Can you work these out from the model? Positions are in its coordinate system, mm. A direction names the side the tool comes from. Give positions to 0.01 mm unless a question says otherwise; leave off trailing zeros. Loops run counter-clockwise (first coordinate to the right, second up) from the corner with the lowest first, then second, coordinate; pieces in that order, holes last. Notation, with made-up numbers: (84.25, 59.5) -> (89.25, 59.5) arc R32 cw to (89.25, 85.5) -> close; hole circle Ø7 at (-12, 28.5). An arc over 180 degrees is marked (long way). Return JSON: item names as keys, results as strings. Group by question number.
Q1. Suppose I cut it at B-B, the plane z = 13. Please give me the cut outline in (x, y).
Q2. Will these pins go through, and if not, where does the flat tip stop? pin 1 (2 mm diameter, centred on x = 10.5, y = 0, fed in from +Z); pin 2 (4 mm diameter, centred on x = 8.5, y = -16.5, fed in from -Z); pin 3 (1.5 mm diameter, centred on x = 3.5, z = 22, fed in from -Y).
Q3. Suppose I cut it at C-C, the plane y = 0. Please give me the cut outline in (x, z), and give its area (3 significant figures).
Q4. Suppose I cut it at A-A, the plane x = 0. Please give me the cut outline in (y, z), and give its area (3 significant figures).
Q5. Which directions (+Z, -Z, +X, -X, +Y, -Y) give clear straight access to the entire face, cutting with the end or side of a thin tool? Please do faces 1 (the flat face through (0, 23, 40)), 2 (the flat face through (0, -22, 25)), 3 (the flat face through (0, -17.5, 17)), 4 (the flat face through (3, 2, 27)).
Q6. I need wall thicknesses on line 1 along Z through (x, y) = (-2.5, 4); line 2 along Z through (x, y) = (14, 11); line 3 along X through (y, z) = (-13.5, 27.5). Which ranges of each line are inside material? Lowest first, please. Write a range as [from, to].
Q7. Suppose I cut it at D-D, the plane z = 44.5. Please give me the cut outline in (x, y).
Q8. Thinking about a two-plate mould opening in Z: for faces 5 (the cylindrical face through (-0.91, -24.01, 51.75)), 6 (the flat face through (0, 0, -5)), 7 (the flat face through (-20, 0, 5)), which applies, pulls with the +Z half, pulls with the -Z half, needs draft (parallel to the pull), parting line crosses it, or undercut?
```python
from build123d import *

# Parameters (mm, degrees)
SKETCH1_W           = 40
SKETCH1_H           = 40
BOSS_EXTRUDE1_DEPTH = 10
BOSS_EXTRUDE2_DEPTH = 15
SKETCH6_W           = 6
SKETCH6_H           = 50
BOSS_EXTRUDE4_DEPTH = 3
SKETCH7_W           = 6
SKETCH7_H           = 2
BOSS_EXTRUDE5_DEPTH = 25
SKETCH8_R           = 1.5
CUT_EXTRUDE1_DEPTH  = 65
SKETCH10_R          = 10
BOSS_EXTRUDE7_DEPTH = 5


with BuildPart() as part:
    # Sketch1 → Boss-Extrude1 (new body)
    with BuildSketch(Plane.XY):
        Rectangle(SKETCH1_W, SKETCH1_H)
    extrude(amount=BOSS_EXTRUDE1_DEPTH)

    # Sketch2 → Boss-Extrude2 (add)
    with BuildSketch(Plane.XY.offset(10)):
        Polygon((0, -20), (3, -20), (3, -17.5), (-3, -17.5), (-3, -20), align=None)
    boss_extrude2 = extrude(amount=BOSS_EXTRUDE2_DEPTH)

    # Mirror1: Boss-Extrude2 across plane
    add(boss_extrude2.mirror(Plane.ZX))

    # Sketch6 → Boss-Extrude4 (add)
    with BuildSketch(Plane.XY.offset(25)):
        Rectangle(SKETCH6_W, SKETCH6_H)
    extrude(amount=BOSS_EXTRUDE4_DEPTH)

    # Sketch7 → Boss-Extrude5 (add)
    with BuildSketch(Plane.XY.offset(28)):
        with Locations((0, -24)):
            Rectangle(SKETCH7_W, SKETCH7_H)
    boss_extrude5 = extrude(amount=BOSS_EXTRUDE5_DEPTH)

    # Mirror2: Boss-Extrude5 across plane
    add(boss_extrude5.mirror(Plane.ZX))

    # Sketch8 → Cut-Extrude1 (cut)
    with BuildSketch(Plane.XZ.offset(25)):
        with Locations(Location((0, 50.555661978, 0), (0, 0, 270))):
            Circle(SKETCH8_R)
    extrude(amount=-CUT_EXTRUDE1_DEPTH, mode=Mode.SUBTRACT)

    # Sketch10 → Boss-Extrude7 (add)
    with BuildSketch(Plane(origin=(0, 0, 0), x_dir=(-1, 0, 0), z_dir=(0, 0, -1))):
        Circle(SKETCH10_R)
    extrude(amount=BOSS_EXTRUDE7_DEPTH)


solid = part.part
```
Ans:
{
 "1": {"outline": "(-3, -20) -> (3, -20) -> (3, -17.5) -> (-3, -17.5) -> close; (-3, 17.5) -> (3, 17.5) -> (3, 20) -> (-3, 20) -> close"},
 "2": {"pin 1": "stops at z = 10", "pin 2": "stops at z = 0", "pin 3": "stops at y = -20"},
 "3": {"outline": "(-20, 0) -> (-10, 0) -> (-10, -5) -> (10, -5) -> (10, 0) -> (20, 0) -> (20, 10) -> (-20, 10) -> close; (-3, 25) -> (3, 25) -> (3, 28) -> (-3, 28) -> close", "area": "518 mm^2"},
 "4": {"outline": "(-25, 25) -> (-20, 25) -> (-20, 0) -> (-10, 0) -> (-10, -5) -> (10, -5) -> (10, 0) -> (20, 0) -> (20, 25) -> (25, 25) -> (25, 49.06) -> (23, 49.06) -> (23, 28) -> (-23, 28) -> (-23, 49.06) -> (-25, 49.06) -> close; (-25, 52.06) -> (-23, 52.06) -> (-23, 53) -> (-25, 53) -> close; (23, 52.06) -> (25, 52.06) -> (25, 53) -> (23, 53) -> close; hole (-17.5, 10) -> (17.5, 10) -> (17.5, 25) -> (-17.5, 25) -> close", "area": "813 mm^2"},
 "5": {"face 1": "+Z, +X, -X", "face 2": "-Z, +X, -X, -Y", "face 3": "+X, -X", "face 4": "+Z, +X, +Y, -Y"},
 "6": {"line 1": "z = [-5, 10], [25, 28]", "line 2": "z = [0, 10]", "line 3": "x = [-3, 3]"},
 "7": {"outline": "(-3, -25) -> (3, -25) -> (3, -23) -> (-3, -23) -> close; (-3, 23) -> (3, 23) -> (3, 25) -> (-3, 25) -> close"},
 "8": {"face 5": "undercut", "face 6": "pulls with the -Z half", "face 7": "needs draft"}
}
